from build123d import *

# Parameters (mm, degrees)
F0_W     = 38.2177424617
F0_H     = 76.4065049589
F1_DEPTH = 50.1015456393
F1_TAPER = -10
F2_R     = 19.05
F3_DEPTH = 25.4


with BuildPart() as f1:
    # F0 (on Top) → F1 (new body, symmetric)
    with BuildSketch(Plane.XY):
        with Locations((19.1088712309, -22.7365922183)):
            Rectangle(F0_W, F0_H)
    extrude(amount=F1_DEPTH, both=True, taper=F1_TAPER)

    # F2 (on face) → F3 (cut)
    with BuildSketch(Plane.XY.offset(50.1015456393)):
        with Locations((25.4, 0)):
            Circle(F2_R)
    extrude(amount=-F3_DEPTH, mode=Mode.SUBTRACT)


solid = f1.part
Build history of the part. All positions in model axes, mm. A direction names the side the tool comes from. Coordinates: 2 decimals unless noted, no trailing zeros. One line per question, with ' | ' between items. Start each with the question number.
Q1. Two-plate mould, pull along Y, no slides. Class faces 3 (the face through (6.37, 0.84, 37.58)), 4 (the face through (19, -24, 50.102)): +Y half, -Y half, draft (parallel to the pull), parting line (faces both ways), or undercut.
Q2. 3-axis set-ups, long thin cutter, end or side, ignore diameter. For faces 1 (the face through (19, -24, -50.102)), 2 (the face through (24, 0, 24.702)): which of +Z, -Z, +X, -X, +Y, -Y reach the whole face in a straight line?
Q3. Probe L1, parallel to Z at x = 33, y = -1.5; L2, parallel to Y at x = 25.4, z = 43; L3, parallel to Y at x = 25, z = 43.5. List the from-to ranges inside material, lowest first. Write a range as from..to.
Q4. Flat gauge pins, fed straight in: pin 1 Ø3 at (y, z) = (1.5, 14.5) entering from +X; pin 2 Ø6 at (x, z) = (33.5, -37.5) entering from -Y; pin 3 Ø6 at (y, z) = (-28, 6.5) entering from +X. Where does each tip first touch, or does it go through?
Check values:
1) face 3: undercut | face 4: draft
2) face 1: -Z, +X, -X, +Y, -Y | face 2: +Z
3) L1: z = -50.1..24.7 | L2: y = -68.52..-19.05, 19.05..23.05 | L3: y = -68.61..-19.05, 19.05..23.14
4) pin 1: stops at x = 41.04 | pin 2: stops at y = -68.08 | pin 3: stops at x = 39.89
